For this review, take the finished solid that the model builds, in its own axes (mm). Round coordinates to 2 decimals unless told otherwise and drop trailing zeros. Write each loop counter-clockwise with the first axis right and the second up, starting at its lowest first coordinate (ties: lowest second). Pieces come first, ordered by that corner, then holes. Notation, with made-up numbers: M 56.5,-23.75 L 64.5,-23.75 A14 ccw 64.5,0.25 Z; hole C 36.5,27 d1. An arc over 180 degrees is marked long. Write each question's results on one line, items separated by ' | '. Start each with the question number.
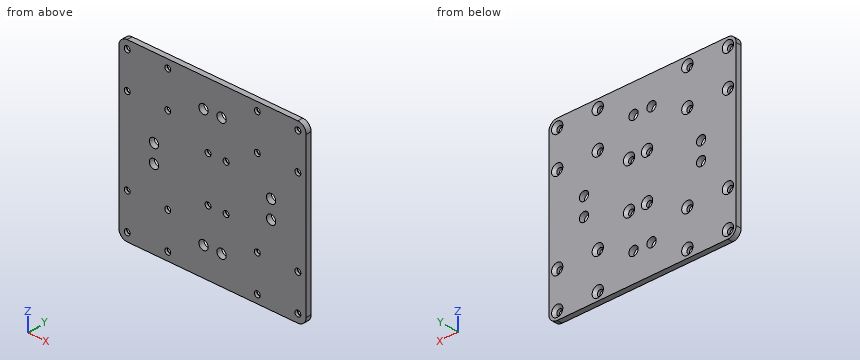
Autodesk Inventor part; units mm, degrees
ref_plane "YZ Plane" through (0, 0, 0) normal (1, 0, 0) x (0, 1, 0)
ref_plane "XZ Plane" through (0, 0, 0) normal (0, 1, 0) x (-1, 0, 0)
ref_plane "XY Plane" through (0, 0, 0) normal (0, 0, 1) x (1, 0, 0)
sketch "Sketch1" plane through (0, 0, 0) normal (0, 1, 0) x (-1, 0, 0)
  circle A0 centre (-12, 20) radius 2.6
  circle A1 centre (4, 20) radius 2.6
  circle A2 centre (4, -20) radius 2.6
  circle A3 centre (-12, -20) radius 2.6
  circle A4 centre (39.75, 38) radius 2.6
  circle A5 centre (39.75, 70) radius 2.6
  circle A6 centre (75.75, 70) radius 2.6
  circle A7 centre (75.75, 38) radius 2.6
  circle A8 centre (39.75, -38) radius 2.6
  circle A9 centre (75.75, -38) radius 2.6
  circle A10 centre (75.75, -70) radius 2.6
  circle A11 centre (39.75, -70) radius 2.6
  circle A12 centre (-39.75, 38) radius 2.6
  circle A13 centre (-39.75, 70) radius 2.6
  circle A14 centre (-75.75, 70) radius 2.6
  circle A15 centre (-75.75, 38) radius 2.6
  circle A16 centre (-39.75, -38) radius 2.6
  circle A17 centre (-39.75, -70) radius 2.6
  circle A18 centre (-75.75, -38) radius 2.6
  circle A19 centre (-75.75, -70) radius 2.6
  line L0 (-78.35, 8) -> (78.35, 8) construction
  line L1 (78.35, 8) -> (78.35, -8) construction
  line L2 (78.35, -8) -> (-78.35, -8) construction
  line L3 (-78.35, -8) -> (-78.35, 8) construction
  line L4 (8, 72.6) -> (-8, 72.6) construction
  line L5 (-8, 72.6) -> (-8, -72.6) construction
  line L6 (-8, -72.6) -> (8, -72.6) construction
  line L7 (8, -72.6) -> (8, 72.6) construction
  circle A20 centre (8, 52) radius 4.1
  line L8 (0, 0) -> (0, 72.6) construction
  line L9 (0, 0) -> (78.35, 0) construction
  circle A21 centre (52, 8) radius 4.1
  circle A22 centre (52, -8) radius 4.1
  circle A23 centre (8, -52) radius 4.1
  circle A24 centre (-8, 52) radius 4.1
  circle A25 centre (-52, 8) radius 4.1
  circle A26 centre (-52, -8) radius 4.1
  circle A27 centre (-8, -52) radius 4.1
  circle A28 centre (75.75, 70) radius 7.3625 construction
  circle A29 centre (75.75, -70) radius 7.3625 construction
  circle A30 centre (-75.75, -70) radius 7.3625 construction
  circle A31 centre (-75.75, 70) radius 7.3625 construction
  line L10 (83.1125, 70) -> (83.1125, -70)
  line L11 (75.75, -77.3625) -> (-75.75, -77.3625)
  line L12 (-83.1125, -70) -> (-83.1125, 70)
  line L13 (-75.75, 77.3625) -> (75.75, 77.3625)
  arc A32 (75.75, -77.3625) -> (83.1125, -70) centre (75.75, -70) ccw
  arc A33 (83.1125, 70) -> (75.75, 77.3625) centre (75.75, 70) ccw
  arc A34 (-75.75, 77.3625) -> (-83.1125, 70) centre (-75.75, 70) ccw
  arc A35 (-83.1125, -70) -> (-75.75, -77.3625) centre (-75.75, -70) ccw
  dimension "d0" = 5.2
  dimension "d1" = 12
  dimension "d2" = 20
  dimension "d3" = 16
  dimension "d4" = 20
  dimension "d5" = 18
  dimension "d6" = 35.75
  dimension "d7" = 32
  dimension "d8" = 36
  dimension "d9" = 18
  dimension "d10" = 32
  dimension "d11" = 27.75
  dimension "d12" = 36
  dimension "d13" = 16
  dimension "d14" = 8
  dimension "d15" = 8
  dimension "d16" = 8.2
  dimension "d18" = 18
  dimension "d20" = 31.75
  dimension "d22" = 30
  dimension "d26" = 4.7625
  dimension "d38" = 8
  dimension "d39" = 8
  dimension "d40" = 8
  dimension "d41" = 52
  dimension "d42" = 52
  dimension "d44" = 52
extrude "Extrusion1" add sketch "Sketch1" along normal blind 4.7625
sketch "Sketch2" plane through (0, 4.7625, 0) normal (0, 1, 0) x (1, 0, 0)
  line L0 (83.1125, -70) -> (83.1125, 70)
  arc A0 (83.1125, 70) -> (75.75, 77.3625) centre (75.75, 70) ccw
  line L1 (75.75, 77.3625) -> (-75.75, 77.3625)
  arc A1 (-75.75, 77.3625) -> (-83.1125, 70) centre (-75.75, 70) ccw
  line L2 (-83.1125, 70) -> (-83.1125, -70)
  arc A2 (-83.1125, -70) -> (-75.75, -77.3625) centre (-75.75, -70) ccw
  line L3 (-75.75, -77.3625) -> (75.75, -77.3625)
  arc A3 (75.75, -77.3625) -> (83.1125, -70) centre (75.75, -70) ccw
  circle A4 centre (8, 52) radius 4.1
  circle A5 centre (8, -52) radius 4.1
  circle A6 centre (-8, 52) radius 4.1
  circle A7 centre (-52, -8) radius 4.1
  circle A8 centre (75.75, 38) radius 2.6
  circle A9 centre (39.75, 38) radius 2.6
  circle A10 centre (39.75, -70) radius 2.6
  circle A11 centre (-39.75, 70) radius 2.6
  circle A12 centre (-39.75, 38) radius 2.6
  circle A13 centre (-75.75, -38) radius 2.6
  circle A14 centre (-39.75, -70) radius 2.6
  circle A15 centre (-39.75, -38) radius 2.6
  circle A16 centre (12, 20) radius 2.6
  circle A17 centre (-4, 20) radius 2.6
  circle A18 centre (-4, -20) radius 2.6
  circle A19 centre (12, -20) radius 2.6
  circle A20 centre (-75.75, 38) radius 2.6
  circle A21 centre (39.75, -38) radius 2.6
  circle A22 centre (75.75, -38) radius 2.6
  circle A23 centre (39.75, 70) radius 2.6
  circle A24 centre (-8, -52) radius 4.1
  circle A25 centre (-52, 8) radius 4.1
  circle A26 centre (52, -8) radius 4.1
  circle A27 centre (52, 8) radius 4.1
  circle A28 centre (75.75, 70) radius 2.6
  circle A29 centre (75.75, -70) radius 2.6
  circle A30 centre (-75.75, 70) radius 2.6
  circle A31 centre (-75.75, -70) radius 2.6
  point P0 (0, 0)
hole "Hole1" at (-75.75, 4.7625, 38) at (-75.75, 4.7625, 70) at (-39.75, 4.7625, 70) at (-39.75, 4.7625, 38) at (-75.75, 4.7625, -38) at (-75.75, 4.7625, -70) at (-39.75, 4.7625, -70) at (-39.75, 4.7625, -38) at (-4, 4.7625, -20) at (12, 4.7625, -20) at (12, 4.7625, 20) at (-4, 4.7625, 20) at (39.75, 4.7625, 38) at (75.75, 4.7625, 38) at (39.75, 4.7625, 70) at (75.75, 4.7625, 70) at (75.75, 4.7625, -38) at (39.75, 4.7625, -38) at (39.75, 4.7625, -70) at (75.75, 4.7625, -70) direction (0, -1, 0) diameter 4.019 end through all countersink diameter 10 countersink angle 90
equation "\"d9\" = d5"
equation "\"d10\" = d7"
equation "\"d12\" = d8"
equation "\"d18\" = 0.5 * d8"
equation "\"d38\" = d39"
equation "\"d40\" = d38"
properties part number "CNC-005-XAxisMount1" material "Steel AISI 1008 91 HR"
Item 1: We need section A-A on z = 8. State the section outline as (x, y) points.
Item 2: We need section C-C on x = -54. State the section outline as (y, z) points.
Item 3: We need section B-B on z = -38. State the section outline as (x, y) points.
Item 4: Insertion check: P1, Ø6, axis at x = 12, z = 20, coming from the +Y side; P2, Ø7, axis at x = 39.75, z = 70, coming from the +Y side; P3, Ø3, axis at x = -75.75, z = -70, coming from the -Y side. Each pin has a flat end and moves straight along its axis. Give the tip position at first contact, or say it passes through.
Item 5: We need section D-D on y = 1.1. State how many separate pieces and enclosed holes the cut face has, then the cut area to 3 significant figures.
Item 6: For probe 1 along Z at (x, y) = (75.75, 1.7); probe 2 along X at (y, z) = (1.55, -20); probe 3 along Z at (x, y) = (-8, 2.05), list the stretches that pass through material, from the lowest coordinate up.
Numbers:
1) outline: M -83.11,0 L -56.1,0 L -56.1,4.76 L -83.11,4.76 Z; M -47.9,0 L 47.9,0 L 47.9,4.76 L -47.9,4.76 Z; M 56.1,0 L 83.11,0 L 83.11,4.76 L 56.1,4.76 Z
2) outline: M 0,-77.36 L 4.76,-77.36 L 4.76,-11.58 L 0,-11.58 Z; M 0,-4.42 L 4.76,-4.42 L 4.76,4.42 L 0,4.42 Z; M 0,11.58 L 4.76,11.58 L 4.76,77.36 L 0,77.36 Z
3) outline: M -83.11,0 L -78.35,0 L -78.35,2.36 L -80.75,4.76 L -83.11,4.76 Z; M -73.15,0 L -42.35,0 L -42.35,2.36 L -44.75,4.76 L -70.75,4.76 L -73.15,2.36 Z; M -37.15,0 L 37.15,0 L 37.15,2.36 L 34.75,4.76 L -34.75,4.76 L -37.15,2.36 Z; M 42.35,0 L 73.15,0 L 73.15,2.36 L 70.75,4.76 L 44.75,4.76 L 42.35,2.36 Z; M 78.35,0 L 83.11,0 L 83.11,4.76 L 80.75,4.76 L 78.35,2.36 Z
4) P1: stops at y = 2.76 | P2: stops at y = 3.26 | P3: passes through
5) separate pieces: 1 | enclosed holes: 28 | area: 24,800 mm^2
6) probe 1: z = -77.36 to -72.6, -67.4 to -40.6, -35.4 to 35.4, 40.6 to 67.4, 72.6 to 77.36 | probe 2: x = -83.11 to -6.6, -1.4 to 9.4, 14.6 to 83.11 | probe 3: z = -77.36 to -56.1, -47.9 to 47.9, 56.1 to 77.36
